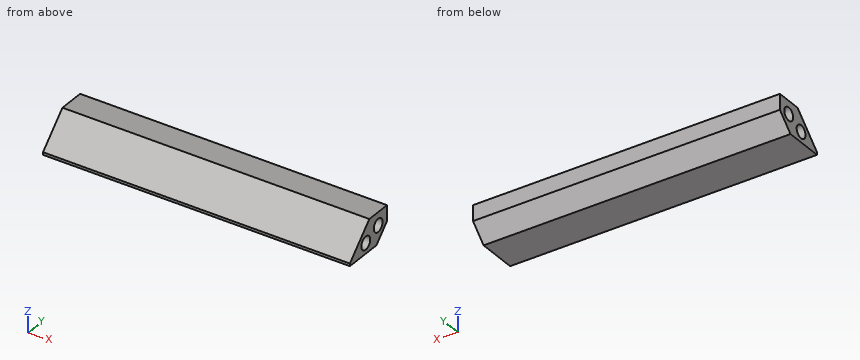
Autodesk Inventor part; units mm, degrees
ref_plane "YZ Plane" through (0, 0, 0) normal (1, 0, 0) x (0, 1, 0)
ref_plane "XZ Plane" through (0, 0, 0) normal (0, 1, 0) x (-1, 0, 0)
ref_plane "XY Plane" through (0, 0, 0) normal (0, 0, 1) x (1, 0, 0)
sketch "Skizze1" plane through (0, 0, 0) normal (1, 0, 0) x (0, 1, 0)
  line L0 (-5, 6) -> (-10.5, 0.5)
  line L1 (-10.5, 0) -> (0, 0)
  line L2 (0, 0) -> (0, 6)
  line L3 (0, 6) -> (-5, 6)
  line L4 (-10.5, 0) -> (-10.5, 0.5)
  dimension "d35" = 45
  dimension "d54" = 6
  dimension "d55" = 0.5
  dimension "d56" = 10.5
extrude "Extrusion1" add sketch "Skizze1" along normal mid plane 59
fillet "Rundung2" [suppressed]
sketch "Skizze5" plane through (29.5, 0, 0) normal (1, 0, 0) x (0, 0, -1)
  line L0 (-7.2, 0) -> (1.2, 0)
  line L1 (0, -12.6) -> (0, 2.1)
  point P0 (0, 0)
  point P1 (-3.7, -4)
  dimension "d36" = 3.7
  dimension "d37" = 4
hole "Bohrung3" [suppressed]
sketch "Skizze6" plane through (29.5, 0, 0) normal (1, 0, 0) x (0, 0, -1)
  line L0 (-7.2, 0) -> (1.2, 0)
  line L1 (0, -12.6) -> (0, 2.1)
  point P0 (0, 0)
  point P1 (-3.5, -2.5)
  point P2 (-2, -6)
  dimension "d45" = 3.5
  dimension "d46" = 2.5
  dimension "d65" = 1.5
  dimension "d66" = 3.5
hole "Bohrung4" at (29.5, -2.5, 3.5) at (29.5, -6, 2) direction (-1, 0, 0) diameter 2.5 depth 6.1 tip angle 118
mirror "Spiegeln1" about plane through (0, 0, 0) normal (1, 0, 0) of "Bohrung4"
sketch "Skizze7" plane through (-29.5, -5, 6) normal (0, 0, 1) x (1, 0, 0)
  line L0 (0, 0) -> (59, 0)
  line L1 (59, 5) -> (59, 0)
  line L2 (59, 5) -> (0, 5)
  line L3 (0, 0) -> (0, 5)
  line L4 (0, 0) -> (0, 5) construction
  line L5 (0, 2.5) -> (59, 2.5) construction
  line L6 (29.5, 5) -> (29.5, 0) construction
  line L7 (0, 0) -> (59, 0) construction
  point P0 (15.5, 2.5)
  point P1 (43.5, 2.5)
  point P2 (29.5, 2.5)
  dimension "d57" = 14
hole "Bohrung5" [suppressed]
chamfer "Fase2" distance 3 angle 45 1 edges at (0, 0, 0)
properties part number "Chip Schaufel Mitte" material "Aluminium 6061"
Can you work these out from the model? Positions are in its coordinate system, mm. Coordinates: 2 decimals unless noted, no trailing zeros. Order: outer loops, then holes, each group sorted by start corner. A loop starts at its lowest first (then second) coordinate and runs counter-clockwise, first axis right, second up. Notation, with made-up numbers: M 2,-12 L 10,-12 A27 ccw 10,23 Z; hole C 88.25,5 d11. An arc over 180 degrees is marked long. Write item = value, one per line.
(1) Suppose I cut it at A-A on x = 20. Please give me the cut outline in (y, z).
Results are:
outline = M -10.5,0 L -3,0 L 0,3 L 0,6 L -5,6 L -10.5,0.5 Z
(2) Suppose I cut it at B-B on y = -9.25. Please give me the cut outline in (x, z).
Results are:
outline = M -29.5,0 L 29.5,0 L 29.5,1.75 L -29.5,1.75 Z
(3) I need wall thicknesses on line 1 along Z through (x, y) = (-26.5, -2.5); line 2 along Y through (x, z) = (-24.75, 2); line 3 along Z through (x, y) = (24.75, -6). Which ranges of each line are inside material? Lowest first, please. Write a range as [from, to].
Results are:
line_1 = [0.5, 2.25], [4.75, 6]
line_2 = [-9, -7.25], [-4.75, -1]
line_3 = [0, 0.75], [3.25, 5]
(4) For pin 1 Ø2 at (y, z) = (-6, 2) entering from -X; pin 2 Ø3 at (y, z) = (-6, 2) entering from -X; pin 3 Ø1.5 at (x, z) = (-0.5, 3.5) entering from -Y; pin 4 Ø2 at (y, z) = (-2.5, 3.5) entering from +X, each with a flat end and sliding along its axis, tell me the tip position at first contact or that it passes through.
Results are:
pin_1 = -23.25
pin_2 = -29.5
pin_3 = -8.25
pin_4 = 23.25
